Here's how the part is built. I have some questions about the finished solid (model axes, mm). A direction names the side the tool comes from. Give positions to 0.01 mm unless a question says otherwise; leave off trailing zeros. Loops run counter-clockwise (first coordinate to the right, second up) from the corner with the lowest first, then second, coordinate; pieces in that order, holes last.
Q1. We'd pull the mould along X, two halves only. Please class faces 1 (the face through (-25.292, -17.01, 1.014)), 2 (the face through (25, 0, 1)), 3 (the face through (0, 0, 0)), 4 (the face through (0, -20, 1)): +X half, -X half, draft (parallel to the pull), parting line (faces both ways), or undercut.
Q2. If we section it at C-C (z = 1.5): Please give me the cut outline in (x, y).
Q3. For faces 5 (the face through (25.31, 17.04, 1.01)), 6 (the face through (-25, 0, 1)), 7 (the face through (-22.04, 20.31, 1.01)), 8 (the face through (-22.04, -20.31, 1.01)), which set-ups out of +Z, -Z, +X, -X, +Y, -Y let a thin tool reach every point of the face, with its end or its side?
Q4. If we section it at B-B (y = 2): Please give me the cut outline in (x, z).
Q5. If we section it at D-D (x = 17.5): Please give me the cut outline in (y, z), plus the area to 3 significant figures.
Q6. I need wall thicknesses on line 1 (Y direction, x = -20.5, z = 0.6); line 2 (Y direction, x = 25.5, z = 0.8); line 3 (X direction, y = -14.5, z = 1.75). Which ranges of each line are inside material? Lowest first, please.
Q7. If we section it at A-A (x = -11.3): Please give me the cut outline in (y, z).
Q8. Will these pins go through, and if not, where does the flat tip stop? P1, Ø0.6, axis at y = 4, z = 1, coming from the +X side; P2, Ø0.6, axis at x = 7.5, z = 0.5, coming from the -Y side; P3, Ø6, axis at x = -11.5, y = 0, coming from the +Z side; P4, Ø1, axis at x = 10, z = 1.5, coming from the +Y side.
from build123d import *

# Parameters (mm, degrees)
F0_R     = 3.5
F1_DEPTH = 2
F3_D     = 3
F4_R     = 2


with BuildPart() as f1:
    # F0 (on Top) → F1 (new body)
    with BuildSketch(Plane.XY):
        with BuildLine():
            Line((-25, 17.5), (-25, 20))
            Line((-25, 20), (-22.5, 20))
            ThreePointArc((-22.5, 20), (-26.767766953, 21.767766953), (-25, 17.5))
        make_face()
        with BuildLine():
            Line((-22.5, 20), (-25, 20))
            Line((-25, 20), (-25, 17.5))
            ThreePointArc((-25, 17.5), (-23.232233047, 18.232233047), (-22.5, 20))
        make_face()
        with BuildLine():
            Line((22.5, 20), (-22.5, 20))
            ThreePointArc((-22.5, 20), (-23.232233047, 18.232233047), (-25, 17.5))
            Line((-25, 17.5), (-25, -17.5))
            ThreePointArc((-25, -17.5), (-23.232233047, -18.232233047), (-22.5, -20))
            Line((-22.5, -20), (22.5, -20))
            ThreePointArc((22.5, -20), (23.232233047, -18.232233047), (25, -17.5))
            Line((25, -17.5), (25, 17.5))
            ThreePointArc((25, 17.5), (23.232233047, 18.232233047), (22.5, 20))
        make_face()
        with Locations((-11.3, 2)):
            Circle(F0_R, mode=Mode.SUBTRACT)
        with BuildLine():
            ThreePointArc((27.5, 20), (25, 22.5), (22.5, 20))
            Line((22.5, 20), (25, 20))
            Line((25, 20), (25, 17.5))
            ThreePointArc((25, 17.5), (26.767766953, 18.232233047), (27.5, 20))
        make_face()
        with BuildLine():
            Line((25, 20), (22.5, 20))
            ThreePointArc((22.5, 20), (23.232233047, 18.232233047), (25, 17.5))
            Line((25, 17.5), (25, 20))
        make_face()
        with BuildLine():
            ThreePointArc((-22.5, -20), (-23.232233047, -18.232233047), (-25, -17.5))
            Line((-25, -17.5), (-25, -20))
            Line((-25, -20), (-22.5, -20))
        make_face()
        with BuildLine():
            Line((-25, -20), (-25, -17.5))
            ThreePointArc((-25, -17.5), (-26.767766953, -21.767766953), (-22.5, -20))
            Line((-22.5, -20), (-25, -20))
        make_face()
        with BuildLine():
            ThreePointArc((27.5, -20), (26.767766953, -18.232233047), (25, -17.5))
            Line((25, -17.5), (25, -20))
            Line((25, -20), (22.5, -20))
            ThreePointArc((22.5, -20), (25, -22.5), (27.5, -20))
        make_face()
        with BuildLine():
            Line((25, -20), (25, -17.5))
            ThreePointArc((25, -17.5), (23.232233047, -18.232233047), (22.5, -20))
            Line((22.5, -20), (25, -20))
        make_face()
    extrude(amount=F1_DEPTH)

    # F3 (through all)
    with Locations(Plane.XY.offset(2)):
        with Locations((-25, 20), (-25, -20), (25, 20), (25, -20)):
            Hole(F3_D / 2)

    # F4
    f4_edges = [f1.edges().sort_by_distance(p)[0] for p in [
        (-25, 17.5, 1),
        (-22.5, 20, 1),
        (22.5, 20, 1),
        (25, 17.5, 1),
        (25, -17.5, 1),
        (22.5, -20, 1),
        (-22.5, -20, 1),
        (-25, -17.5, 1),
    ]]
    fillet(f4_edges, radius=F4_R)


solid = f1.part
Check sheet entries:
1. face 1: -X half
1. face 2: +X half
1. face 3: draft
1. face 4: undercut
2. outline: (-26.11, -17.76) arc R2.5 ccw (long way) to (-22.76, -21.11) arc R2 cw to (-20.97, -20) - (20.97, -20) arc R2 cw to (22.76, -21.11) arc R2.5 ccw (long way) to (26.11, -17.76) arc R2 cw to (25, -15.97) - (25, 15.97) arc R2 cw to (26.11, 17.76) arc R2.5 ccw (long way) to (22.76, 21.11) arc R2 cw to (20.97, 20) - (-20.97, 20) arc R2 cw to (-22.76, 21.11) arc R2.5 ccw (long way) to (-26.11, 17.76) arc R2 cw to (-25, 15.97) - (-25, -15.97) arc R2 cw to start; hole circle Ø3 at (-25, -20); hole circle Ø3 at (-25, 20); hole circle Ø7 at (-11.3, 2); hole circle Ø3 at (25, -20); hole circle Ø3 at (25, 20)
3. face 5: +Z, -Z, +X
3. face 6: +Z, -Z, -X
3. face 7: +Z, -Z, +Y
3. face 8: +Z, -Z, -Y
4. outline: (-25, 0) - (-14.8, 0) - (-14.8, 2) - (-25, 2) - close; (-7.8, 0) - (25, 0) - (25, 2) - (-7.8, 2) - close
5. outline: (-20, 0) - (20, 0) - (20, 2) - (-20, 2) - close
5. area: 80.0 mm2
6. line 1: y = -20 to 20
6. line 2: y = -22.45 to -21.41, -18.59 to -17.29, 17.29 to 18.59, 21.41 to 22.45
6. line 3: x = -25 to 25
7. outline: (-20, 0) - (-1.5, 0) - (-1.5, 2) - (-20, 2) - close; (5.5, 0) - (20, 0) - (20, 2) - (5.5, 2) - close
8. P1: stops at x = 25
8. P2: stops at y = -20
8. P3: stops at z = 2
8. P4: stops at y = 20
